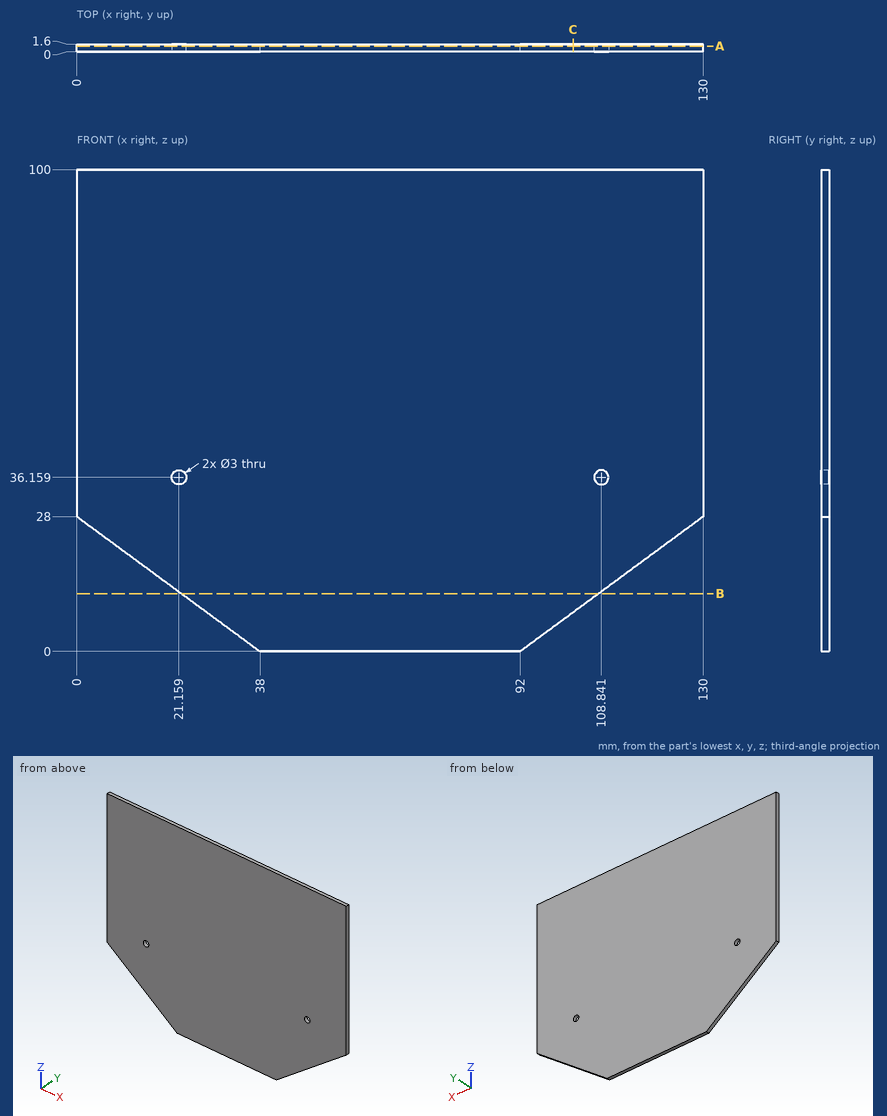
Geometry: see drawing. Coordinates: mm, zero at the bounding-box minimum. Coordinates: 2 decimals unless noted, no trailing zeros. Write each loop counter-clockwise with the first axis right and the second up, starting at its lowest first coordinate (ties: lowest second). Pieces come first, ordered by that corner, then holes. Notation, with made-up numbers: M -37,76.25 L -12,76.25 A30 cw -12,100.25 Z; hole C -27,-32 d10. An arc over 180 degrees is marked long. Answer as a JSON object with one key per item and string values.
1. Contact query for a flat-ended pin moving along its axis: P1, Ø8, axis at x = 102, z = 15.5, coming from the -Y side. Output: stop coordinate, or through.
Evaluation:
{"P1": "y = 0"}
2. Cut plane B-B on z = 12. Output: boundary loops of the cut face in (x, y) (1 decimal).
Evaluation:
{"outline": "M 21.7,0 L 108.3,0 L 108.3,1.6 L 21.7,1.6 Z"}
3. Cut plane C-C on x = 103. Output: boundary loops of the cut face in (y, z) (1 decimal).
Evaluation:
{"outline": "M 0,8.1 L 1.6,8.1 L 1.6,100 L 0,100 Z"}
4. Cut plane A-A on y = 1.15. Output: boundary loops of the cut face in (x, z), plus the area to 3 significant figures.
Evaluation:
{"outline": "M 0,28 L 38,0 L 92,0 L 130,28 L 130,100 L 0,100 Z; hole C 21.16,36.16 d3; hole C 108.84,36.16 d3", "area": "11,900 mm^2"}
5. Ray query, L1, parallel to X at y = 0.15, z = 35 (1 decimal); L2, parallel to Z at x = 108, y = 0.6; L3, parallel to Z at x = 35, y = 0.75. Return the intervals inside material, ascending.
Evaluation:
{"L1": "0 to 20.2, 22.1 to 107.9, 109.8 to 130", "L2": "11.79 to 34.92, 37.4 to 100", "L3": "2.21 to 100"}
